```python
from build123d import *

# Parameters (mm, degrees)
FILLET1_R = 0.6


with BuildPart() as part:
    # Sketch1 → Revolve1 (revolve)
    with BuildSketch(Plane.XY, mode=Mode.PRIVATE) as revolve1_sk:
        Polygon((-81.066688046, 0), (81.066688046, 0), (81.066688046, 32.5325), (40.066688046, 32.5325), (22.066688046, 32.5325), (22.066688046, 33), (-15.469523763, 33), (-57.066688046, 33), (-57.066688046, 38), (-62.066688046, 38), (-62.066688046, 22.5225), (-81.066688046, 22.5225), align=None)
    revolve(revolve1_sk.sketch.rotate(Axis((-122.765721942, 0, 0), (1, 0, 0)), 180), axis=Axis((-122.765721942, 0, 0), (1, 0, 0)))

    # Fillet1
    # the kernel refuses this fillet: 0.6 mm, written as the material it adds along each edge
    with BuildSketch(Plane(origin=(22.066688046, 0, 0), x_dir=(0, -1, 0), z_dir=(0, 0, 1))) as fillet1_piece_1:
        with BuildLine():
            CenterArc((33.1325, 0.585186936), FILLET1_R, 180, 77.242016626)
            Line((33, 0), (32.99735, -0.011703739))
            ThreePointArc((32.99735, -0.011703739), (32.76625, -0.012), (32.5325, -0.012))
            Line((32.5325, -0.012), (32.5205, 0))
            Line((32.5205, 0), (32.5205, 0.585186936))
            Line((32.5205, 0.585186936), (32.5325, 0.585186936))
        make_face()
    revolve(axis=Axis((22.066688046, 0, 0), (1, 0, 0)))
    with BuildSketch(Plane(origin=(-57.066688046, 0, 0), x_dir=(0, -1, 0), z_dir=(0, 0, 1))) as fillet1_piece_2:
        with BuildLine():
            CenterArc((33 + FILLET1_R, FILLET1_R), FILLET1_R, 180, 90)
            Line((33 + FILLET1_R, 0), (33 + FILLET1_R, -FILLET1_R * 0.02))
            Line((33 + FILLET1_R, -FILLET1_R * 0.02), (33 - FILLET1_R * 0.02, -FILLET1_R * 0.02))
            Line((33 - FILLET1_R * 0.02, -FILLET1_R * 0.02), (33 - FILLET1_R * 0.02, FILLET1_R))
            Line((33 - FILLET1_R * 0.02, FILLET1_R), (33, FILLET1_R))
        make_face()
    revolve(axis=Axis((-57.066688046, 0, 0), (1, 0, 0)))
    with BuildSketch(Plane(origin=(-62.066688046, 0, 0), x_dir=(0, -1, 0), z_dir=(0, 0, 1))) as fillet1_piece_3:
        with BuildLine():
            CenterArc((22.5225 + FILLET1_R, -FILLET1_R), FILLET1_R, 90, 90)
            Line((22.5225, -FILLET1_R), (22.5225 - FILLET1_R * 0.02, -FILLET1_R))
            Line((22.5225 - FILLET1_R * 0.02, -FILLET1_R), (22.5225 - FILLET1_R * 0.02, FILLET1_R * 0.02))
            Line((22.5225 - FILLET1_R * 0.02, FILLET1_R * 0.02), (22.5225 + FILLET1_R, FILLET1_R * 0.02))
            Line((22.5225 + FILLET1_R, FILLET1_R * 0.02), (22.5225 + FILLET1_R, 0))
        make_face()
    revolve(axis=Axis((-62.066688046, 0, 0), (1, 0, 0)))


solid = part.part
```
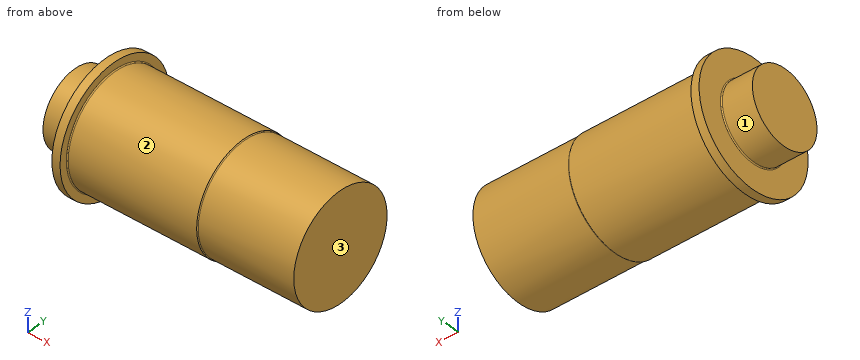
Design review of the part built by this model. Coordinates are the model's own, in mm. Face numbers are marked on the shaded views. A direction names the side the tool comes from. Give positions to 0.01 mm unless a question says otherwise; leave off trailing zeros. Write each loop counter-clockwise with the first axis right and the second up, starting at its lowest first coordinate (ties: lowest second). Pieces come first, ordered by that corner, then holes. Notation, with made-up numbers: (37.5, -4) - (78.5, -4) arc R6 ccw to (78.5, 7) - close; hole circle Ø3 at (21.25, -20.75). An arc over 180 degrees is marked (long way). Return JSON: item names as keys, results as strings. Group by question number.
(1) We need section D-D, the plane x = -67.5. Give the boundary of the cut face in (y, z) (1 decimal), then the cut area to 3 significant figures.
(2) To check wall thickness, follow probe 1 along X at (y, z) = (29, -9); probe 2 along X at (y, z) = (26, 21); probe 3 along Y at (x, z) = (19, 1). State the ranges of each line that lie inside material, in increasing order.
(3) Insertion check: pin 1 (12 mm diameter, centred on x = -56, y = -10.5, fed in from +Z); pin 2 (6 mm diameter, centred on x = 0, z = -22, fed in from -Y); pin 3 (3 mm diameter, centred on x = -35.5, y = -14.5, fed in from -Z). Each pin has a flat end and moves straight along its axis. Give the tip position at first contact, or say it passes through.
(4) We need section A-A, the plane z = 0. Give the boundary of the cut face in (x, y), then the cut area to 3 significant figures.
(5) We need section C-C, the plane x = 30.5. Give the boundary of the cut face in (y, z) (1 decimal).
(6) Machinability: for the marked faces 1, 2 and 3, which of the approach directions +Z, -Z, +X, -X, +Y, -Y give a long, thin tool a straight path to every point of the face, cutting with its end or side? Answer none if there is none.
Reported:
{
 "1": {"outline": "circle Ø45 at (0, 0)", "area": "1,590 mm2"},
 "2": {"probe 1": "x = -62.07 to 81.07", "probe 2": "x = -62.07 to -57.04", "probe 3": "y = -32.98 to 32.98"},
 "3": {"pin 1": "stops at z = 37.72", "pin 2": "stops at y = -26.98", "pin 3": "stops at z = -30.33"},
 "4": {"outline": "(-81.07, -22.52) - (-62.67, -22.52) arc R0.6 cw to (-62.07, -23.12) - (-62.07, -38) - (-57.07, -38) - (-57.07, -33.6) arc R0.6 cw to (-56.47, -33) - (22.07, -33) arc R0.6 cw to (22.65, -32.53) - (81.07, -32.53) - (81.07, 32.53) - (22.65, 32.53) arc R0.6 cw to (22.07, 33) - (-56.47, 33) arc R0.6 cw to (-57.07, 33.6) - (-57.07, 38) - (-62.07, 38) - (-62.07, 23.12) arc R0.6 cw to (-62.67, 22.52) - (-81.07, 22.52) - close", "area": "10,300 mm2"},
 "5": {"outline": "circle Ø65.1 at (0, 0)"},
 "6": {"face 1": "-X", "face 2": "+X", "face 3": "+Z, -Z, +X, +Y, -Y"}
}
